```python
from build123d import *

# Parameters (mm, degrees)
SKETCH1_W                      = 11.9
SKETCH1_H                      = 11.9
BOSS_EXTRUDE1_DEPTH            = 29
CUT_EXTRUDE1_REACH             = 13.9
SKETCH2_R                      = 4.05
CUT_EXTRUDE1_DIRECTION_2_DEPTH = 1
SKETCH3_R                      = 12.5
BOSS_EXTRUDE2_DEPTH            = 3.5


with BuildPart() as part:
    # Sketch1 → Boss-Extrude1 (new body)
    with BuildSketch(Plane(origin=(0, 0, 0), x_dir=(0, 0, -1), z_dir=(1, 0, 0))):
        Rectangle(SKETCH1_W, SKETCH1_H)
    extrude(amount=BOSS_EXTRUDE1_DEPTH)

    # Sketch2 → Cut-Extrude1 (cut, up to next)
    with BuildSketch(Plane.XY.offset(5.95), mode=Mode.PRIVATE) as cut_extrude1_sk1:
        with Locations((15, 0)):
            Circle(SKETCH2_R)
    cut_extrude1_tool1 = extrude(cut_extrude1_sk1.sketch, amount=-CUT_EXTRUDE1_REACH, mode=Mode.PRIVATE) & part.part
    add(cut_extrude1_tool1.solids().sort_by_distance((15, 0, 5.95))[0], mode=Mode.SUBTRACT)

    # Sketch2 → Cut-Extrude1 direction 2 (cut)
    with BuildSketch(Plane.XY.offset(5.95)):
        with Locations((15, 0)):
            Circle(SKETCH2_R)
    extrude(amount=CUT_EXTRUDE1_DIRECTION_2_DEPTH, mode=Mode.SUBTRACT)

    # Sketch3 → Boss-Extrude2 (add)
    with BuildSketch(Plane.ZY):
        Circle(SKETCH3_R)
    extrude(amount=BOSS_EXTRUDE2_DEPTH)

    # Sketch4 → Revolve1 (revolve)
    with BuildSketch(Plane.XY):
        Polygon((-3.5, 0), (-3.5, 12.5), (-25.150635095, 0), align=None)
    revolve(axis=Axis((0, 0, 0), (-1, 0, 0)))


solid = part.part
```
The model under review builds one solid part; all positions refer to its coordinate system, in mm. A direction names the side the tool comes from. Give positions to 0.01 mm unless a question says otherwise; leave off trailing zeros. Write each loop counter-clockwise with the first axis right and the second up, starting at its lowest first coordinate (ties: lowest second). Pieces come first, ordered by that corner, then holes.
(1) Consider section B-B, the plane x = -1. Give the boundary of the cut face in (y, z).
(2) To check wall thickness, follow L1, parallel to Y at x = 15, z = -3; L2, parallel to Z at x = 8, y = 1.25; L3, parallel to X at y = 7.75, z = 5.75. State the ranges of each line that lie inside material, in increasing order.
(3) Consider section A-A, the plane x = 15. Give the boundary of the cut face in (y, z).
(4) Tool access review of faces 1 (the flat face through (11, -3, 5.95)), 2 (the flat face through (14, 5.95, 0)), 3 (the flat face through (11, -3, -5.95)): name each direction out of +Z, -Z, +X, -X, +Y, -Y from which nothing blocks a thin tool from reaching the whole face with its end or side.
(5) For P1, Ø6, axis at x = -6.5, z = 1, coming from the -Y side; P2, Ø9.5, axis at x = 10, z = 3, coming from the -Y side; P3, Ø9.5, axis at x = 11.5, y = -1, coming from the +Z side, all flat-tipped, find the tip position at first contact; note any pin that passes through.
(6) Consider section C-C, the plane x = -16.5. Give the boundary of the cut face in (y, z), and give its area (3 significant figures).
(7) The part is to be moulded in two halves that separate along Y. For faces 4 (the cylindrical face through (10.954, 0.178, 0.083)), 5 (the flat face through (14, -5.95, 0)), 6 (the conical face through (-16.882, -1.035, 4.66)), say which applies: released by +Y, released by -Y, zero draft, split by the parting line, or undercut.
Returned:
1. outline: circle Ø25 at (0, 0)
2. L1: y = -5.95 to -4.05, 4.05 to 5.95
2. L2: z = -5.95 to 5.95
2. L3: x = -8.44 to 0
3. outline: (-5.95, -5.95) - (-4.05, -5.95) - (-4.05, 5.95) - (-5.95, 5.95) - close; (4.05, -5.95) - (5.95, -5.95) - (5.95, 5.95) - (4.05, 5.95) - close
4. face 1: +Z, +X, +Y, -Y
4. face 2: +Z, -Z, +X, +Y
4. face 3: -Z, +X, +Y, -Y
5. P1: stops at y = -12.47
5. P2: stops at y = -5.95
5. P3: stops at z = 5.95
6. outline: circle Ø9.99 at (0, 0)
6. area: 78.4 mm2
7. face 4: undercut
7. face 5: released by -Y
7. face 6: split by the parting line
